Here's the drawing with two shaded views (mm, measured from the low corner). I have some questions. Give positions to 0.01 mm unless a question says otherwise; leave off trailing zeros. Write each loop counter-clockwise with the first axis right and the second up, starting at its lowest first coordinate (ties: lowest second). Pieces come first, ordered by that corner, then holes. Notation, with made-up numbers: (-7, 50.5) - (43, 50.5) arc R22 cw to (43, 73.5) - close; hole circle Ø8 at (-31.75, -1). An arc over 180 degrees is marked (long way). Write item = value, one per line.
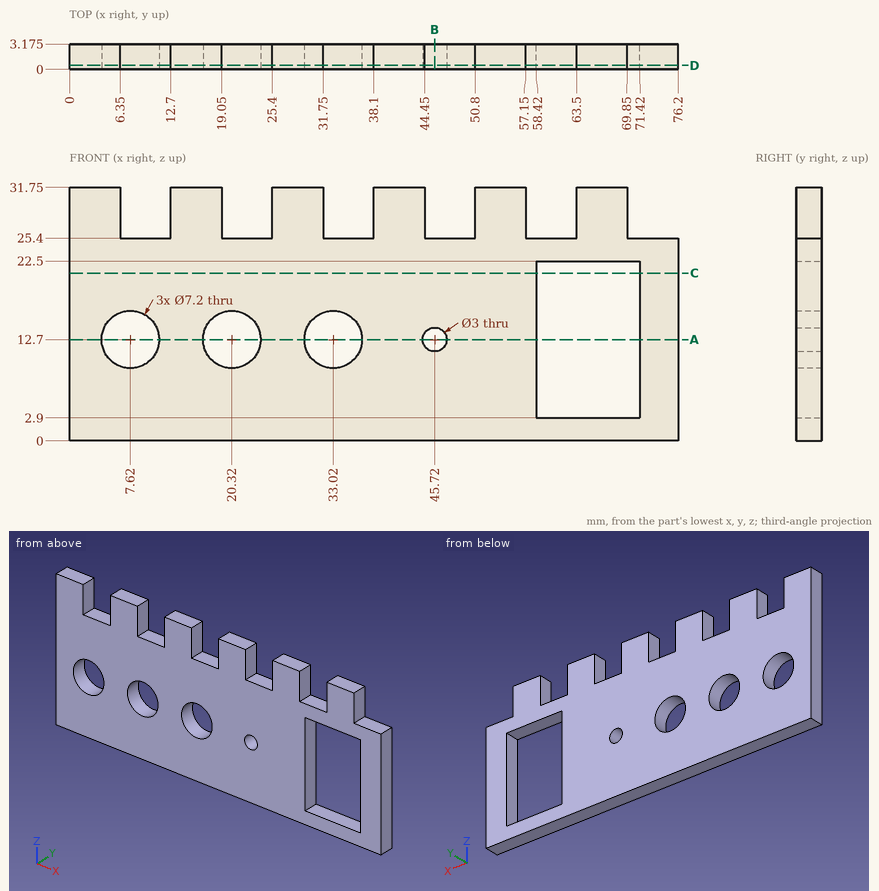
1. If we section it at A-A, the plane z = 12.7: Please give me the cut outline in (x, y) (3 decimals), and give its area (3 significant figures).
Filled sheet:
outline = (0, 0) - (4.02, 0) - (4.02, 3.175) - (0, 3.175) - close; (11.22, 0) - (16.72, 0) - (16.72, 3.175) - (11.22, 3.175) - close; (23.92, 0) - (29.42, 0) - (29.42, 3.175) - (23.92, 3.175) - close; (36.62, 0) - (44.22, 0) - (44.22, 3.175) - (36.62, 3.175) - close; (47.22, 0) - (58.42, 0) - (58.42, 3.175) - (47.22, 3.175) - close; (71.42, 0) - (76.2, 0) - (76.2, 3.175) - (71.42, 3.175) - close
area = 123 mm2
2. If we section it at C-C, the plane z = 21: Please give me the cut outline in (x, y) (3 decimals).
Filled sheet:
outline = (0, 0) - (58.42, 0) - (58.42, 3.175) - (0, 3.175) - close; (71.42, 0) - (76.2, 0) - (76.2, 3.175) - (71.42, 3.175) - close
3. If we section it at B-B, the plane x = 45.72: Please give me the cut outline in (y, z) (3 decimals), and give its area (3 significant figures).
Filled sheet:
outline = (0, 0) - (3.175, 0) - (3.175, 11.2) - (0, 11.2) - close; (0, 14.2) - (3.175, 14.2) - (3.175, 25.4) - (0, 25.4) - close
area = 71.1 mm2
4. I need wall thicknesses on line 1 (X direction, y = 2.2, z = 12.7); line 2 (X direction, y = 1.65, z = 27); line 3 (X direction, y = 0.5, z = 5). Which ranges of each line are inside material? Lowest first, please.
Filled sheet:
line_1 = 0 to 4.02, 11.22 to 16.72, 23.92 to 29.42, 36.62 to 44.22, 47.22 to 58.42, 71.42 to 76.2
line_2 = 0 to 6.35, 12.7 to 19.05, 25.4 to 31.75, 38.1 to 44.45, 50.8 to 57.15, 63.5 to 69.85
line_3 = 0 to 58.42, 71.42 to 76.2
5. For pin 1 (1 mm diameter, centred on x = 22.5, y = 1, fed in from +Z); pin 2 (1 mm diameter, centred on y = 1.5, z = 30, fed in from +X), each with a flat end and sliding along its axis, tell me the tip position at first contact or that it passes through.
Filled sheet:
pin_1 = 25.4
pin_2 = 69.85
6. If we section it at D-D, the plane y = 0.5: Count the separate pieces of the cut face and the enclosed holes in it, and give its area (3 significant figures).
Filled sheet:
separate_pieces = 1
enclosed_holes = 5
area = 1,790 mm2
